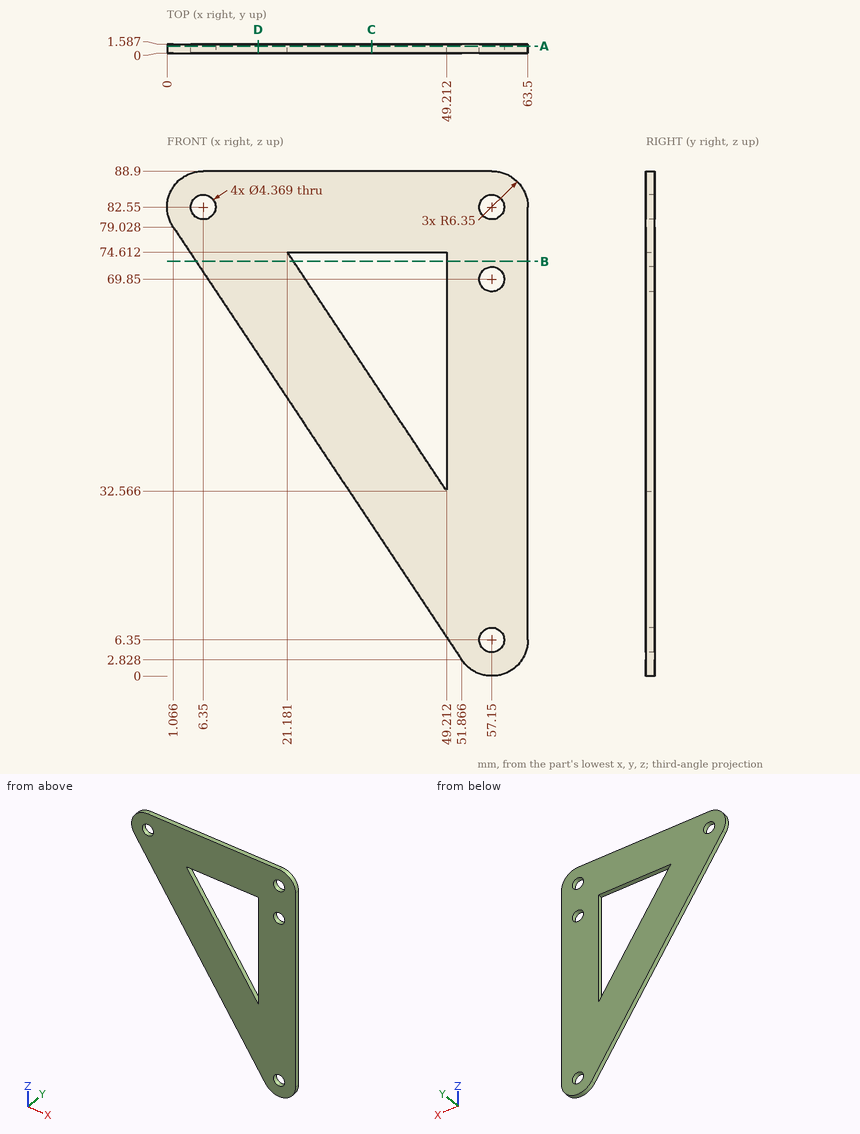
For this review, use the dimensioned drawing (mm, ordinates from the lowest corner) and the shaded views. Round coordinates to 2 decimals unless told otherwise and drop trailing zeros. Write each loop counter-clockwise with the first axis right and the second up, starting at its lowest first coordinate (ties: lowest second). Pieces come first, ordered by that corner, then holes. Notation, with made-up numbers: (-8, -28) - (2, -28) arc R14 ccw to (2, -12) - close; hole circle Ø6 at (-31, 79). An arc over 180 degrees is marked (long way). Answer as a JSON object with one key per item and string values.
1. We need section C-C on x = 36. Give the boundary of the cut face in (y, z) (1 decimal).
Response values:
{"outline": "(0, 26.6) - (1.6, 26.6) - (1.6, 52.4) - (0, 52.4) - close; (0, 74.6) - (1.6, 74.6) - (1.6, 88.9) - (0, 88.9) - close"}
2. We need section D-D on x = 16. Give the boundary of the cut face in (y, z).
Response values:
{"outline": "(0, 56.63) - (1.59, 56.63) - (1.59, 88.9) - (0, 88.9) - close"}
3. We need section B-B on z = 73. Give the boundary of the cut face in (x, y) (1 decimal).
Response values:
{"outline": "(5.1, 0) - (22.3, 0) - (22.3, 1.6) - (5.1, 1.6) - close; (49.2, 0) - (63.5, 0) - (63.5, 1.6) - (49.2, 1.6) - close"}
4. For pin 1 Ø5.5 at (x, z) = (57.15, 82.55) entering from -Y; pin 2 Ø4 at (x, z) = (57.15, 69.85) entering from -Y; pin 3 Ø0.5 at (y, z) = (1, 46) entering from -X; pin 4 Ø0.8 at (x, y) = (37, 1) entering from -Z (1 decimal), all flat-tipped, find the tip position at first contact; note any pin that passes through.
Response values:
{"pin 1": "stops at y = 0", "pin 2": "passes through", "pin 3": "stops at x = 22.92", "pin 4": "stops at z = 24.5"}
5. To check wall thickness, follow line 1 along X through (y, z) = (0.45, 69.5) (1 decimal); line 2 along Z through (x, y) = (34, 0.9) (1 decimal); line 3 along X through (y, z) = (0.15, 47.5) (1 decimal). State the ranges of each line that lie inside material, in increasing order.
Response values:
{"line 1": "x = 7.4 to 24.6, 49.2 to 55, 59.3 to 63.5", "line 2": "z = 29.6 to 55.4, 74.6 to 88.9", "line 3": "x = 22.1 to 39.3, 49.2 to 63.5"}
6. We need section A-A on y = 1.2. Count the separate pieces of the cut face and the enclosed holes in it, then the cut area to 3 significant figures.
Response values:
{"separate pieces": "1", "enclosed holes": "5", "area": "2,800 mm2"}
